Geometry: final body of the model. Coordinates: model frame, mm. A direction names the side the tool comes from. Give positions to 0.01 mm unless a question says otherwise; leave off trailing zeros. Write each loop counter-clockwise with the first axis right and the second up, starting at its lowest first coordinate (ties: lowest second). Pieces come first, ordered by that corner, then holes.
Q1. Section D-D (z = -67). Return the cut outline in (x, y).
Q2. Line query: line 1 (X direction, y = 20, z = -59); line 2 (Y direction, x = 1, z = -30); line 3 (Y direction, x = 30, z = -50.5). Output: solid intervals per line, ascending.
Q3. Reachability of faces 4 (the flat face through (1, 19, -90)), 5 (the flat face through (35, 0, -59)), 6 (the flat face through (3, 23, -46)) from +Z, -Z, +X, -X, +Y, -Y: full face, straight path, thin tool, end or side. Return the list, or none.
Q4. Section B-B (y = 59.5). Return the cut outline in (x, z).
Q5. Section C-C (x = 44). Return the cut outline in (y, z), plus the area to 3 significant figures.
Q6. Section A-A (z = -30). Return the cut outline in (x, y), plus the area to 3 significant figures.
Q7. Pin query (flat end, axial travel): pin 1 Ø1 at (x, z) = (21.5, -34) entering from +Y; pin 2 Ø3.5 at (x, y) = (68, 33.5) entering from -Z; pin 3 Ø2.5 at (x, z) = (68.5, -93.5) entering from +Y. Return the tip coordinate at first contact, or that it passes through.
Q8. Mould query, pull axis X, two halves, no side actions, for faces 1 (the cylindrical face through (68.48, 22.42, -63.61)), 2 (the flat face through (70, 26, -46)), 3 (the cylindrical face through (25.166, 1.521, -101.714)). Classes: +X half, -X half, draft (parallel to the pull), parting line (faces both ways), or undercut.
Autodesk Inventor part; units mm, degrees
ref_plane "YZ Plane" through (0, 0, 0) normal (1, 0, 0) x (0, 1, 0)
ref_plane "XZ Plane" through (0, 0, 0) normal (0, 1, 0) x (-1, 0, 0)
ref_plane "XY Plane" through (0, 0, 0) normal (0, 0, 1) x (1, 0, 0)
sketch "Sketch1" plane through (0, 0, 0) normal (0, 1, 0) x (-1, 0, 0)
  line L0 (0, 0) -> (-70, 0)
  line L1 (-70, 0) -> (-70, -120)
  line L2 (-70, -120) -> (0, -120)
  line L3 (0, -120) -> (0, 0)
  line L4 (0, -120) -> (-3, -120)
  line L5 (-3, -120) -> (-3, 0)
  line L6 (-70, 0) -> (-67, 0)
  line L7 (-67, 0) -> (-67, -120)
  dimension "d0" = 70
  dimension "d1" = 120
  dimension "d2" = 3
  dimension "d3" = 3
extrude "Extrusion1" add sketch "Sketch1" along normal blind 3
sketch "Sketch2" plane through (0, 3, 0) normal (0, 1, 0) x (1, 0, 0)
  line L0 (70, 0) -> (70, 120)
  line L1 (70, 120) -> (0, 120)
  line L2 (0, 120) -> (0, 0)
  line L3 (0, 0) -> (70, 0)
  line L4 (70, 0) -> (70, 120)
  line L5 (70, 120) -> (67, 120)
  line L6 (67, 120) -> (67, 0)
  line L7 (0, 0) -> (3, 0)
  line L8 (3, 0) -> (3, 120)
  dimension "d6" = 3
  dimension "d7" = 3
extrude "Extrusion2" add sketch "Sketch2" along normal blind 70 contours L3 L6 L1 L0 | L3 L2 L1 L8
sketch "Sketch3" plane through (0, 0, -120) normal (-1, 0, 0) x (0, 0, 1)
  line L0 (120, 0) -> (90, 0)
  line L1 (90, 0) -> (120, 0)
  line L2 (90, 0) -> (127, 0)
  line L3 (120, 0) -> (0, 0)
  line L4 (90, 0) -> (90, 37)
  circle A0 centre (90, 37) radius 18
  circle A1 centre (90, 37) radius 30
  line L5 (0, 0) -> (0, 7)
  line L6 (0, 3) -> (0, 73)
  line L7 (12, 19) -> (48, 19)
  arc A2 (12, 19) -> (0, 7) centre (12, 7) ccw
  line L8 (60, 37) -> (60, 31)
  arc A3 (48, 19) -> (60, 31) centre (48, 31) ccw
  line L9 (0, 7) -> (0, 73)
  line L10 (0, 73) -> (120, 73)
  line L11 (120, 73) -> (120, 37)
  point P0 (0, 19)
  point P1 (66, 19)
  dimension "d10" = 30
  dimension "d12" = 37
  dimension "d13" = 36
  dimension "d14" = 60
  dimension "d15" = 19
  dimension "d16" = 12
  dimension "d17" = 12
extrude "Extrusion3" cut sketch "Sketch3" against normal blind 70 contours L8 A3 L7 A2 L6 L10 L11 A1
sketch "Sketch4" plane through (0, 0, -120) normal (-1, 0, 0) x (0, 0, 1)
  line L0 (120, 0) -> (90, 0)
  line L1 (0, 0) -> (120, 0)
  line L2 (90, 0) -> (90, 37)
  circle A0 centre (90, 37) radius 18
  dimension "d20" = 30
  dimension "d21" = 37
  dimension "d22" = 36
extrude "Extrusion4" cut sketch "Sketch4" against normal blind 70
fillet "Fillet1" radius 3 2 edges at (3, 3, -60) (67, 3, -60)
sketch "Sketch5" plane through (0, 3, 0) normal (0, 1, 0) x (1, 0, 0)
  line L0 (67, 0) -> (67, 120)
  line L1 (67, 120) -> (56, 120)
  line L2 (70, 120) -> (0, 120)
  line L3 (3, 120) -> (3, 0)
  line L4 (3, 120) -> (5.3284, 120)
  line L5 (3, 120) -> (14, 120)
  circle A0 centre (48.0638, 86.1207) radius 7
  circle A1 centre (48.0638, 107.9241) radius 7
  circle A2 centre (21.9362, 86.1207) radius 7
  circle A3 centre (21.9362, 107.9241) radius 7
  point P0 (0, 0)
extrude "Extrusion5" cut sketch "Sketch5" against normal blind 70
properties part number "whateverthisis"
Computed:
1. outline: (0, 0) - (70, 0) - (70, 20.09) - (67, 20.09) - (67, 6) arc R3 cw to (64, 3) - (6, 3) arc R3 cw to (3, 6) - (3, 20.09) - (0, 20.09) - close
2. line 1: x = 0 to 3, 67 to 70
2. line 2: y = 0 to 19, 55 to 67
2. line 3: y = 0 to 3
3. face 4: -Z, +X, -X, +Y
3. face 5: +Z, -Z, +X, -X, -Y
3. face 6: +Z, -Z, +Y
4. outline: (0, -49.84) - (3, -49.84) - (3, -10.16) - (0, -10.16) - close; (67, -49.84) - (70, -49.84) - (70, -10.16) - (67, -10.16) - close
5. outline: (0, -120) - (3, -120) - (3, -113.62) - (0, -113.62) - close; (0, -102.22) - (3, -102.22) - (3, -91.82) - (0, -91.82) - close; (0, -80.42) - (3, -80.42) - (3, 0) - (0, 0) - close
5. area: 292 mm2
6. outline: (0, 0) - (70, 0) - (70, 19) - (67, 19) - (67, 6) arc R3 cw to (64, 3) - (6, 3) arc R3 cw to (3, 6) - (3, 19) - (0, 19) - close; (0, 55) - (3, 55) - (3, 67) - (0, 67) - close; (67, 55) - (70, 55) - (70, 67) - (67, 67) - close
6. area: 382 mm2
7. pin 1: stops at y = 3
7. pin 2: stops at z = -60
7. pin 3: stops at y = 19
8. face 1: draft
8. face 2: +X half
8. face 3: undercut
